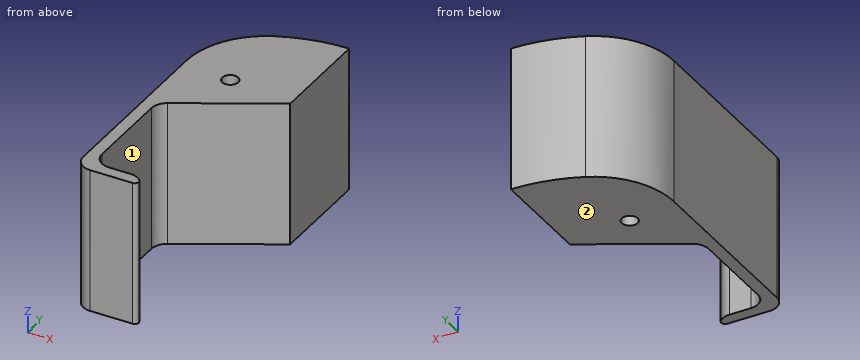
Autodesk Inventor part; units mm, degrees
ref_plane "YZ Plane" through (0, 0, 0) normal (1, 0, 0) x (0, 1, 0)
ref_plane "XZ Plane" through (0, 0, 0) normal (0, 1, 0) x (-1, 0, 0)
ref_plane "XY Plane" through (0, 0, 0) normal (0, 0, 1) x (1, 0, 0)
sketch "Schizzo1" plane through (0, 0, 0) normal (0, 0, 1) x (1, 0, 0)
  line L0 (9.6257, 10.2674) -> (9.6257, -2.6852)
  arc A0 (9.6257, 10.2674) -> (-4.5165, 4.4095) centre (9.6257, -9.7326) ccw
  line L1 (-0.3743, -9.7326) -> (-4.5165, 4.4095) construction
  line L2 (9.6257, 0.2674) -> (-4.5165, 4.4095) construction
  line L3 (4.6257, -4.7326) -> (9.6257, 0.2674) construction
  line L4 (-4.5165, 4.4095) -> (4.6257, -4.7326) construction
  line L5 (9.6257, 0.2674) -> (-2.4454, -2.6616) construction
  circle A1 centre (1.5783, -1.6852) radius 1
  line L6 (-4.5165, 4.4095) -> (-4.5165, -25.2326)
  line L7 (-4.5165, -25.2326) -> (-3.0165, -25.2326)
  line L8 (-3.0165, -23.7326) -> (-3.0165, -9.7326)
  line L9 (-3.0165, -25.2326) -> (3.5901, -25.2326)
  line L10 (3.5901, -25.2326) -> (3.5901, -23.7326)
  line L11 (3.5901, -23.7326) -> (-3.0165, -23.7326)
  line L12 (-3.0165, -9.7326) -> (9.6257, -2.6852)
  point P0 (0, 0)
  dimension "d6" = 2
  dimension "d24" = 1.5
  dimension "d27" = 14
  dimension "d28" = 1.5
extrude "Estrusione1" add sketch "Schizzo1" along normal blind 18
fillet "Raccordo11" radius 2 4 edges at (-3.0165, -9.7326, 9) (-3.0165, -23.7326, 9) (-4.5165, -25.2326, 9) (3.5901, -23.7326, 9)
fillet "Raccordo12" radius 10 1 edges at (-4.5165, 4.4095, 9)
fillet "Raccordo13" radius 0.5 1 edges at (3.5901, -25.2326, 9)
properties part number "Gancio1" material "Plastica ABS"
Could you check a few things on this model? Use its own coordinates, in mm. Face numbers are marked on the shaded views. A direction names the side the tool comes from. Give positions to 0.01 mm unless a question says otherwise; leave off trailing zeros. Loops run counter-clockwise (first coordinate to the right, second up) from the corner with the lowest first, then second, coordinate; pieces in that order, holes last. Notation, with made-up numbers: (24.25, 80) -> (77.25, 80) arc R20 cw to (77.25, 106) -> close; hole circle Ø10 at (42, 74.5). An arc over 180 degrees is marked (long way). Put each result on its own line as item: value.
(1) Imagine slicing it at A-A on x = -0.25. Write out the boundary of the cut face in (y, z), plus the area to 3 significant figures.
Computed:
outline: (-25.23, 0) -> (-23.73, 0) -> (-23.73, 18) -> (-25.23, 18) -> close; (-8.19, 0) -> (7.56, 0) -> (7.56, 18) -> (-8.19, 18) -> close
area: 311 mm^2
(2) For the marked faces 1 and 2, which set-ups out of +Z, -Z, +X, -X, +Y, -Y let a thin tool reach every point of the face, with its end or its side?
Computed:
face 1: +Z, -Z, +X
face 2: -Z, +X, -X, +Y, -Y
(3) I'm going to push flat-ended pins straight in: pin 1 Ø8.5 at (y, z) = (-15.5, 11.5) entering from +X; pin 2 Ø3 at (x, z) = (-1, 5.5) entering from +Y; pin 3 Ø8 at (x, z) = (5, 6.5) entering from +Y; pin 4 Ø2.5 at (x, y) = (1.58, -1.69) entering from -Z. Where does each tip first touch, or does it pass through?
Computed:
pin 1: x = -3.02
pin 2: y = 8.04
pin 3: y = 10.26
pin 4: z = 0
(4) Please list where these lines run through material, in increasing order: probe 1 along Y at (x, z) = (-2.25, 7.5); probe 2 along X at (y, z) = (-14.5, 4); probe 3 along Y at (x, z) = (-2, 13.5). Write a range as [from, to].
Computed:
probe 1: [-25.23, -23.31], [-9.33, 5.71]
probe 2: [-4.52, -3.02]
probe 3: [-25.23, -23.47], [-9.17, 6]
(5) Imagine slicing it at B-B on z = 6.5. Write out the boundary of the cut face in (x, y), plus the area to 3 significant figures.
Computed:
outline: (-4.52, -23.23) arc R2 ccw to (-2.52, -25.23) -> (2.77, -25.23) arc R0.5 ccw to (3.14, -24.4) arc R2 ccw to (1.65, -23.73) -> (-1.02, -23.73) arc R2 cw to (-3.02, -21.73) -> (-3.02, -10.91) arc R2 cw to (-1.99, -9.16) -> (9.63, -2.69) -> (9.63, 10.27) arc R20 ccw to (1.34, 8.47) arc R10 ccw to (-4.52, -0.63) -> close; hole circle Ø2 at (1.58, -1.69)
area: 237 mm^2
(6) Imagine slicing it at D-D on x = 4. Write out the boundary of the cut face in (y, z).
Computed:
outline: (-5.82, 0) -> (9.46, 0) -> (9.46, 18) -> (-5.82, 18) -> close
(7) Imagine slicing it at C-C on y = -11.5. Write out the boundary of the cut face in (x, z).
Computed:
outline: (-4.52, 0) -> (-3.02, 0) -> (-3.02, 18) -> (-4.52, 18) -> close
